Geometry: final body of the model. Coordinates: model frame, mm. Face numbers are marked on the shaded views. A direction names the side the tool comes from. Round coordinates to 2 decimals unless told otherwise and drop trailing zeros. Loops run counter-clockwise (first coordinate to the right, second up) from the corner with the lowest first, then second, coordinate; pieces in that order, holes last. Notation, with made-up numbers: (-8.5, 28) -> (-0.5, 28) arc R12 ccw to (-0.5, 48) -> close; hole circle Ø4 at (-15.5, 55). An arc over 180 degrees is marked (long way). Answer in a Markdown table with one row per item.
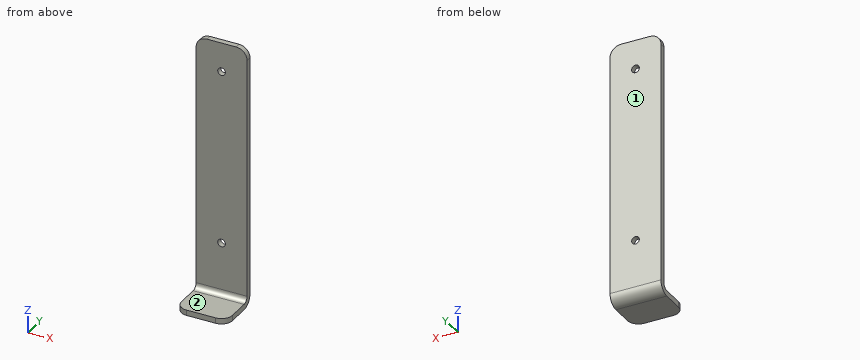
```python
from build123d import *

# Parameters (mm, degrees)
BOSS_EXTRUDE1_DEPTH = 44.45
FILLET1_R           = 4.7752
FILLET2_R           = 9.525
FILLET3_R           = 9.525
SKETCH2_R           = 3.3655
CUT_EXTRUDE1_DEPTH  = 39.1


with BuildPart() as part:
    # Sketch1 → Boss-Extrude1 (new body)
    with BuildSketch(Plane(origin=(0, 0, 0), x_dir=(0, 0, -1), z_dir=(1, 0, 0))):
        Polygon((0, 0), (0, 33.3248), (-223.8248, 33.3248), (-223.8248, 38.1), (4.7752, 38.1), (4.7752, 0), align=None)
    extrude(amount=BOSS_EXTRUDE1_DEPTH)

    # Fillet1
    fillet1_edges = [part.edges().sort_by_distance(p)[0] for p in [
        (22.225, 33.3248, 0),
    ]]
    fillet(fillet1_edges, radius=FILLET1_R)

    # Fillet2
    fillet2_edges = [part.edges().sort_by_distance(p)[0] for p in [
        (22.225, 38.1, -4.7752),
    ]]
    fillet(fillet2_edges, radius=FILLET2_R)

    # Fillet3
    fillet3_edges = [part.edges().sort_by_distance(p)[0] for p in [
        (44.45, 35.7124, 223.8248),
        (44.45, 0, -2.3876),
        (0, 35.7124, 223.8248),
        (0, 0, -2.3876),
    ]]
    fillet(fillet3_edges, radius=FILLET3_R)

    # Sketch2 → Cut-Extrude1 (cut, through all)
    with BuildSketch(Plane(origin=(0, 38.1, 0), x_dir=(1, 0, 0), z_dir=(0, 1, 0))):
        with Locations((22.225, -198.4248)):
            Circle(SKETCH2_R)
        with Locations((22.225, -46.0248)):
            Circle(SKETCH2_R)
    extrude(amount=-CUT_EXTRUDE1_DEPTH, mode=Mode.SUBTRACT)


solid = part.part
```
Item 1: Section query B-B, the plane z = 69. Output: boundary loops of the cut face in (x, y).
Ans:
| item | result |
|---|---|
| outline | (0, 33.32) -> (44.45, 33.32) -> (44.45, 38.1) -> (0, 38.1) -> close |
Item 2: Section query D-D, the plane y = 21. Output: boundary loops of the cut face in (x, z).
Ans:
| item | result |
|---|---|
| outline | (0, -4.78) -> (44.45, -4.78) -> (44.45, 0) -> (0, 0) -> close |
Item 3: Ray query, L1, parallel to Y at x = 5.5, z = 157; L2, parallel to Z at x = 6.5, y = 15.5; L3, parallel to Z at x = 15.5, y = 35.5. Return the intervals inside material, ascending.
Ans:
| item | result |
|---|---|
| L1 | 33.32 to 38.1 |
| L2 | -4.78 to 0 |
| L3 | -1.79 to 223.82 |
Item 4: First-contact query: P1, Ø5.5, axis at x = 22.22, z = 198.42, coming from the +Y side; P2, Ø6, axis at x = 22.5, y = 16, coming from the +Z side; P3, Ø12, axis at x = 9, z = 135.5, coming from the -Y side. Flat tips, straight axial feed; report the tip coordinate or a pass-through.
Ans:
| item | result |
|---|---|
| P1 | through |
| P2 | z = 0 |
| P3 | y = 33.32 |
Item 5: Section query A-A, the plane x = 23. Output: boundary loops of the cut face in (y, z) (3 decimals), and give its area (3 significant figures).
Ans:
| item | result |
|---|---|
| outline | (0, -4.775) -> (28.575, -4.775) arc R9.525 ccw to (38.1, 4.75) -> (38.1, 42.75) -> (33.325, 42.75) -> (33.325, 4.775) arc R4.775 cw to (28.55, 0) -> (0, 0) -> close; (33.325, 49.3) -> (38.1, 49.3) -> (38.1, 195.15) -> (33.325, 195.15) -> close; (33.325, 201.7) -> (38.1, 201.7) -> (38.1, 223.825) -> (33.325, 223.825) -> close |
| area | 1,170 mm2 |
Item 6: Section query C-C, the plane x = 42. Output: boundary loops of the cut face in (y, z) (3 decimals), and give its area (3 significant figures).
Ans:
| item | result |
|---|---|
| outline | (3.148, -4.775) -> (28.575, -4.775) arc R9.525 ccw to (38.1, 4.75) -> (38.1, 220.677) -> (33.325, 220.677) -> (33.325, 4.775) arc R4.775 cw to (28.55, 0) -> (3.148, 0) -> close |
| area | 1,210 mm2 |
Item 7: Set-up query: the marked faces 1 and 2. Return all of +Z, -Z, +X, -X, +Y, -Y with unobstructed straight access to the full face (end or side cutting, diameter ignored); none if empty.
Ans:
| item | result |
|---|---|
| face 1 | +Z, -Z, +X, -X, +Y |
| face 2 | +Z, +X, -X, -Y |
